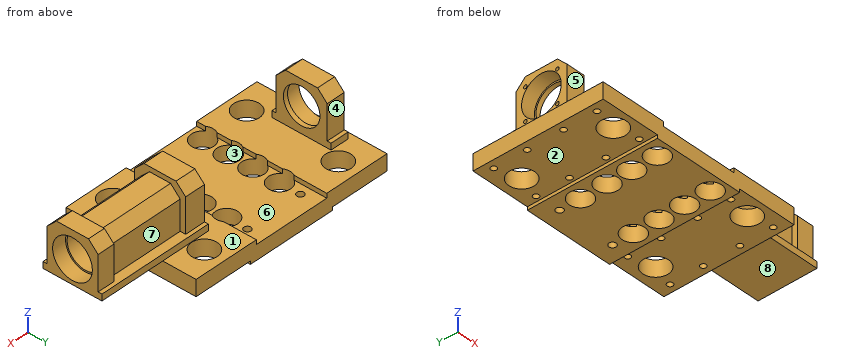
```python
from build123d import *

# Parameters (mm, degrees)
F1_DEPTH  = 203
F4_DEPTH  = 29
F5_SIZE   = 15
F6_R      = 28.5
F7_DEPTH  = 7
F8_R      = 31
F9_DEPTH  = 22
F11_D     = 9
F11_DEPTH = 22
F11_TIP   = 2.7038727856
F12_D     = 40
F14_D     = 35
F15_D     = 11
F18_R     = 31
F19_DEPTH = 32
F20_SIZE  = 15
F21_R     = 31
F22_DEPTH = 122
F23_SIZE  = 15
F24_R     = 31
F25_DEPTH = 27
F26_SIZE  = 15
F28_D     = 5.5
F28_DEPTH = 10
F28_TIP   = 1.6523667023
F29_R     = 31
F30_DEPTH = 181
F31_R     = 31
F32_DEPTH = 5
F33_DEPTH = 27
F34_R     = 28.5
F35_DEPTH = 154
F36_R     = 31
F36_R_2   = 28.5
F37_DEPTH = 22


with BuildPart() as f1:
    # F0 (on Front) → F1 (new body)
    with BuildSketch(Plane.XZ):
        Polygon((0, 25), (0, 0), (92.5, 0), (92.5, -5), (232.5, -5), (232.5, 0), (325, 0), (325, 25), (222.5, 25), (222.5, 18), (102.5, 18), (102.5, 25), align=None)
    extrude(amount=-F1_DEPTH)

    # F3 (on offset) → F4 (join)
    with BuildSketch(Plane.YZ.offset(38.5)):
        Polygon((59, 25), (151, 25), (151, 35), (145, 35), (145, 104), (65, 104), (65, 35), (59, 35), align=None)
    extrude(amount=-F4_DEPTH)

    # F5
    f5_edges = [f1.edges().sort_by_distance(p)[0] for p in [
        (24, 65, 104),
        (24, 145, 104),
    ]]
    chamfer(f5_edges, length=F5_SIZE)

    # F6 (on face) → F7 (cut)
    with BuildSketch(Plane.YZ.offset(38.5)):
        with Locations((105.1451787353, 65)):
            Circle(F6_R)
    extrude(amount=-F7_DEPTH, mode=Mode.SUBTRACT)

    # F8 (on face) → F9 (cut)
    with BuildSketch(Plane(origin=(9.5, 0, 0), x_dir=(0, -1, 0), z_dir=(-1, 0, 0))):
        with Locations((-105, 65)):
            Circle(F8_R)
    extrude(amount=-F9_DEPTH, mode=Mode.SUBTRACT)

    # F11
    with Locations(Plane(origin=(0, 0, 0), x_dir=(1, 0, 0), z_dir=(0, 0, -1))):
        with Locations((12.5, -182), (12.5, -130), (12.5, -73), (12.5, -21), (84.5, -73), (84.5, -130), (84.5, -182), (240.5, -182), (312.5, -182), (240.5, -130), (312.5, -130), (240.5, -73), (312.5, -73), (240.5, -21), (312.5, -21), (84.5, -21)):
            Hole(F11_D / 2, depth=F11_DEPTH)
            with Locations((0, 0, -(F11_DEPTH + F11_TIP / 2))):  # 118° drill point
                Cone(0, F11_D / 2, F11_TIP, mode=Mode.SUBTRACT)

    # F12 (through all)
    with Locations(Plane(origin=(0, 0, 0), x_dir=(1, 0, 0), z_dir=(0, 0, -1))):
        with Locations((48.5, -28.5), (48.5, -171.5), (276.5, -28.5), (276.5, -171.5)):
            Hole(F12_D / 2)

    # F14 (through all)
    with Locations(Plane(origin=(0, 0, -5), x_dir=(1, 0, 0), z_dir=(0, 0, -1))):
        with Locations((117.5, -23), (117.5, -63), (117.5, -143), (207.5, -143), (207.5, -103), (117.5, -101.5), (207.5, -63), (207.5, -23)):
            Hole(F14_D / 2)

    # F15 (through all)
    with Locations(Plane(origin=(0, 0, -5), x_dir=(1, 0, 0), z_dir=(0, 0, -1))):
        with Locations((117.5, -175.5), (207.5, -175.5)):
            Hole(F15_D / 2)

    # F18 (on offset) → F19 (join)
    with BuildSketch(Plane.YZ.offset(247.5)):
        Polygon((59, 25), (151, 25), (151, 35), (145, 35), (145, 104), (65, 104), (65, 35), (59, 35), align=None)
        with Locations((105.1451787353, 65)):
            Circle(F18_R, mode=Mode.SUBTRACT)
    extrude(amount=F19_DEPTH)

    # F20
    f20_edges = [f1.edges().sort_by_distance(p)[0] for p in [
        (263.5, 65, 104),
        (263.5, 145, 104),
    ]]
    chamfer(f20_edges, length=F20_SIZE)

    # F21 (on face) → F22 (join)
    with BuildSketch(Plane.YZ.offset(279.5)):
        Polygon((151, 35), (145, 35), (136.5, 35), (136.5, 96.5), (73.5, 96.5), (73.5, 35), (65, 35), (59, 35), (59, 25), (151, 25), align=None)
        with Locations((105.1451787353, 65)):
            Circle(F21_R, mode=Mode.SUBTRACT)
    extrude(amount=F22_DEPTH)

    # F23
    f23_edges = [f1.edges().sort_by_distance(p)[0] for p in [
        (340.5, 73.5, 96.5),
        (340.5, 136.5, 96.5),
    ]]
    chamfer(f23_edges, length=F23_SIZE)

    # F24 (on face) → F25 (join)
    with BuildSketch(Plane.YZ.offset(401.5)):
        Polygon((65, 104), (65, 35), (73.5, 35), (73.5, 81.5), (88.5, 96.5), (121.5, 96.5), (136.5, 81.5), (136.5, 35), (145, 35), (145, 104), align=None)
        Polygon((59, 35), (59, 25), (151, 25), (151, 35), (145, 35), (136.5, 35), (136.5, 81.5), (121.5, 96.5), (88.5, 96.5), (73.5, 81.5), (73.5, 35), (65, 35), align=None)
        with Locations((105.1451787353, 65)):
            Circle(F24_R, mode=Mode.SUBTRACT)
    extrude(amount=F25_DEPTH)

    # F26
    f26_edges = [f1.edges().sort_by_distance(p)[0] for p in [
        (415, 65, 104),
        (415, 145, 104),
    ]]
    chamfer(f26_edges, length=F26_SIZE)

    # F28
    with Locations(Plane(origin=(9.5, 0, 0), x_dir=(0, -1, 0), z_dir=(-1, 0, 0))):
        with Locations((-130, 89.5), (-80, 89.5), (-130, 39.5), (-80, 39.5)):
            Hole(F28_D / 2, depth=F28_DEPTH)
            with Locations((0, 0, -(F28_DEPTH + F28_TIP / 2))):  # 118° drill point
                Cone(0, F28_D / 2, F28_TIP, mode=Mode.SUBTRACT)

    # F29 (on face) → F30 (join)
    with BuildSketch(Plane.YZ.offset(428.5)):
        with Locations((105.1451787353, 65)):
            Circle(F29_R)
    extrude(amount=-F30_DEPTH)

    # F31 (on face) → F32 (join)
    with BuildSketch(Plane(origin=(247.5, 0, 0), x_dir=(0, -1, 0), z_dir=(-1, 0, 0))):
        with Locations((-105, 62)):
            Circle(F31_R)
    extrude(amount=-F32_DEPTH)

    # F31 (on face) → F33 (cut)
    with BuildSketch(Plane(origin=(247.5, 0, 0), x_dir=(0, -1, 0), z_dir=(-1, 0, 0))):
        with Locations((-105, 62)):
            Circle(F31_R)
    extrude(amount=-F33_DEPTH, mode=Mode.SUBTRACT)

    # F34 (on face) → F35 (cut)
    with BuildSketch(Plane.YZ.offset(428.5)):
        with Locations((105, 62)):
            Circle(F34_R)
    extrude(amount=-F35_DEPTH, mode=Mode.SUBTRACT)

    # F36 (on face) → F37 (cut)
    with BuildSketch(Plane.YZ.offset(428.5)):
        with Locations((105, 62)):
            Circle(F36_R)
        with Locations((105, 62)):
            Circle(F36_R_2, mode=Mode.SUBTRACT)
    extrude(amount=-F37_DEPTH, mode=Mode.SUBTRACT)


solid = f1.part
```
Can you work these out from the model? Positions are in its coordinate system, mm. Face numbers are marked on the shaded views. A direction names the side the tool comes from. Coordinates: 2 decimals unless noted, no trailing zeros. Loops run counter-clockwise (first coordinate to the right, second up) from the corner with the lowest first, then second, coordinate; pieces in that order, holes last. Notation, with made-up numbers: (69.25, 38) -> (99.25, 38) arc R26 ccw to (99.25, 67) -> close; hole circle Ø3 at (26, -35). An arc over 180 degrees is marked (long way). Put each result on its own line as item: value. Start each with the question number.
Q1. Thinking about a two-plate mould opening in X: for the marked faces 1, 2 and 3, which applies, pulls with the +X half, pulls with the -X half, needs draft (parallel to the pull), parting line crosses it, or undercut?
Q2. I want a section at C-C (x = 177). Write out the boundary of the cut face in (y, z).
Q3. For the marked faces 4, 5, 6, 7 and 8, which set-ups out of +Z, -Z, +X, -X, +Y, -Y let a thin tool reach every point of the face, with its end or its side?
Q4. I want a section at B-B (x = 45). Write out the boundary of the cut face in (y, z), plus the area to 3 significant figures.
Q5. If I drill on line 1 (Y direction, x = 84, z = 8); line 2 (X direction, y = 144.5, z = 52); line 3 (X direction, y = 101.5, z = 12.5), over which ranges is the centre line in solid material (lowest first)? Write a range as [from, to].
Q6. I'm going to push flat-ended pins straight in: P1, Ø1, axis at x = 364, y = 97.5, coming from the -Z side; P2, Ø8, axis at y = 144, z = 61.5, coming from the -X side; P3, Ø1, axis at x = 352.5, y = 118, coming from the +Z side; P4, Ø2, axis at y = 132, z = 67, coming from the -X side. Where does each tip first touch, or does it pass through?
Q7. I want a section at A-A (z = 7). Count the separate pieces of the cut face and the enclosed holes in it, plus the area to 3 significant figures.
Taken from the geometry:
1. face 1: undercut
1. face 2: needs draft
1. face 3: undercut
2. outline: (0, -5) -> (203, -5) -> (203, 18) -> (0, 18) -> close
3. face 4: +Z, +X, -X, +Y
3. face 5: +Z, +X, -X, -Y
3. face 6: +Z, +Y, -Y
3. face 7: +Z, +Y
3. face 8: -Z, +X, +Y, -Y
4. outline: (0, 0) -> (8.81, 0) -> (8.81, 25) -> (0, 25) -> close; (48.19, 0) -> (151.81, 0) -> (151.81, 25) -> (48.19, 25) -> close; (191.19, 0) -> (203, 0) -> (203, 25) -> (191.19, 25) -> close
4. area: 3,110 mm2
5. line 1: y = [0, 16.53], [25.47, 68.53], [77.47, 125.53], [134.47, 177.53], [186.47, 203]
5. line 2: x = [9.5, 38.5], [247.5, 279.5], [401.5, 428.5]
5. line 3: x = [0, 100], [135, 190.06], [224.94, 325]
6. P1: stops at z = 25
6. P2: stops at x = 9.5
6. P3: stops at z = 96.5
6. P4: passes through
7. separate pieces: 1
7. enclosed holes: 30
7. area: 52,000 mm2
